Input: part model. Units: mm. Frame: model coordinates. A direction names the side the tool comes from. Give positions to 0.01 mm unless a question says otherwise; leave off trailing zeros. Loops run counter-clockwise (first coordinate to the right, second up) from the corner with the lowest first, then second, coordinate; pieces in that order, holes last. Notation, with made-up numbers: M 6,66 L 54,66 A24 cw 54,78 Z; hole C -13,45.5 d3. An arc over 180 degrees is marked long. Use a Markdown table: item, result. Add a question column.
from build123d import *

# Parameters (mm, degrees)
SKETCH_1_R      = 2.1
EXTRUDE_1_DEPTH = 17.45
SKETCH_2_R      = 4.15
EXTRUDE_2_DEPTH = 3.5
SKETCH_3_R      = 4.15
EXTRUDE_3_DEPTH = 3.5
FILLET_1_R      = 1.5


with BuildPart() as part:
    # ｽｹｯﾁ1 → ﾎﾞｽ - 押し出し1 (new body)
    with BuildSketch(Plane.XY):
        Polygon((-5, -13.5), (5, -13.5), (8.5, -10), (24.6, -10), (24.6, 10), (-24.6, 10), (-24.6, -10), (-8.5, -10), align=None)
        with Locations((-12.7, -4.3)):
            Circle(SKETCH_1_R, mode=Mode.SUBTRACT)
        with Locations(Location((12.7, -4.3, 0), (0, 0, 180))):
            Circle(SKETCH_1_R, mode=Mode.SUBTRACT)
    extrude(amount=EXTRUDE_1_DEPTH)

    # ｽｹｯﾁ2 → ﾎﾞｽ - 押し出し2 (add)
    with BuildSketch(Plane.XZ.offset(10)):
        with Locations(Location((-20, 8.725, 0), (0, 0, 180))):
            Circle(SKETCH_2_R)
        with Locations(Location((20, 8.725, 0), (0, 0, 180))):
            Circle(SKETCH_2_R)
    extrude(amount=EXTRUDE_2_DEPTH)

    # ｽｹｯﾁ3 → ﾎﾞｽ - 押し出し3 (add)
    with BuildSketch(Plane.XZ.offset(13.5)):
        with Locations(Location((0, 8.725, 0), (0, 0, 180))):
            Circle(SKETCH_3_R)
    extrude(amount=EXTRUDE_3_DEPTH)

    # ｽｹｯﾁ5 → 回転1 (revolve)
    with BuildSketch(Plane.XY.offset(8.725)):
        with BuildLine():
            Line((-10.6, 10), (-18.6, 10))
            Line((-18.6, 10), (-18.6, 12))
            Line((-18.6, 12), (-16.6, 12))
            Line((-16.6, 12), (-16.6, 25))
            Line((-16.6, 25), (-14.75, 25))
            Line((-14.75, 25), (-14.75, 31.78842818))
            ThreePointArc((-14.75, 31.78842818), (-15, 32.03842818), (-14.75, 32.28842818))
            Line((-14.75, 32.28842818), (-14.75, 34))
            ThreePointArc((-14.75, 34), (-12.680005458, 34.216234269), (-10.6, 34.28842818))
            Line((-10.6, 34.28842818), (-10.6, 34))
            Line((-10.6, 34), (-10.6, 10))
        make_face()
    revolve(axis=Axis((-10.6, 27.136449726, 8.725), (0, -1, 0)))

    # ﾌｨﾚｯﾄ1
    fillet_1_edges = [part.edges().sort_by_distance(p)[0] for p in [
        (24.6, 0, 17.45),
        (-24.6, 0, 17.45),
        (-24.6, 0, 0),
        (24.6, 0, 0),
    ]]
    fillet(fillet_1_edges, radius=FILLET_1_R)


solid = part.part
1) Contact query for flat-ended pins moving along their axis: P1, Ø1, axis at x = 13.5, z = 8, coming from the -Y side; P2, Ø6.5, axis at x = -21.5, z = 9, coming from the -Y side; P3, Ø3, axis at x = 8, z = 8, coming from the -Y side. Output: stop coordinate, or through.
2) Section query B-B, the plane y = -4.3. Return the cut outline in (x, z), and give its area (3 significant figures).
3) Ray query, line 1 (Y direction, x = -12.7, z = 4.25); line 2 (X direction, y = -12, z = 6.5); line 3 (X direction, y = -13, z = 7.5). Return the intervals inside material, ascending. Write a range as [from, to].
4) Reachability of faces 1 (the cylindrical face through (-6.454, 28.442, 8.543)), 2 (the flat face through (-20, -13.5, 9)), 3 (the flat face through (-14, 12, 3)) from +Z, -Z, +X, -X, +Y, -Y: full face, straight path, thin tool, end or side. Return the list, or none.
5) Section query D-D, the plane z = 14. Return the cut outline in (x, y).
6) Section query C-C, the plane x = -20. Return the cut outline in (y, z) (3 decimals), and give its area (3 significant figures).
7) Section query A-A, the plane x = 12.7. Return the cut outline in (y, z), and give its area (3 significant figures).
8) Pull-direction query (X, two-part tool) for faces 4 (the flat face through (6.7, -11.8, 8.6)), 5 (the flat face through (24.6, 0, 9)), 6 (the cylindrical face through (-9.819, 18.591, 2.776)); classes: pulls with the +X half, pulls with the -X half, needs draft (parallel to the pull), parting line crosses it, or undercut.
Entries:
| question | item | result |
|---|---|---|
| 1 | P1 | stops at y = -10 |
| 1 | P2 | stops at y = -13.5 |
| 1 | P3 | stops at y = -12 |
| 2 | outline | M -24.6,1.5 A1.5 ccw -23.1,0 L -14.8,0 L -14.8,17.45 L -23.1,17.45 A1.5 ccw -24.6,15.95 Z; M -10.6,0 L 10.6,0 L 10.6,17.45 L -10.6,17.45 Z; M 14.8,0 L 23.1,0 A1.5 ccw 24.6,1.5 L 24.6,15.95 A1.5 ccw 23.1,17.45 L 14.8,17.45 Z |
| 2 | area | 710 mm² |
| 3 | line 1 | y = [-10, -6.4], [-2.2, 25] |
| 3 | line 2 | x = [-23.5, -16.5], [-6.5, 6.5], [16.5, 23.5] |
| 3 | line 3 | x = [-23.97, -16.03], [-5.5, 5.5], [16.03, 23.97] |
| 4 | face 1 | none |
| 4 | face 2 | +Z, -Z, -X, -Y |
| 4 | face 3 | +Y |
| 5 | outline | M -24.6,-10 L -8.5,-10 L -5,-13.5 L 5,-13.5 L 8.5,-10 L 24.6,-10 L 24.6,10 L -4.59,10 L -4.59,12 L -7.74,12 L -7.74,25 L -13.46,25 L -13.46,12 L -16.61,12 L -16.61,10 L -24.6,10 Z; hole C -12.7,-4.3 d4.2; hole C 12.7,-4.3 d4.2 |
| 6 | outline | M -13.5,4.575 L -10,4.575 L -10,0 L 10,0 L 10,17.45 L -10,17.45 L -10,12.875 L -13.5,12.875 Z |
| 6 | area | 378 mm² |
| 7 | outline | M -10,0 L -6.4,0 L -6.4,17.45 L -10,17.45 Z; M -2.2,0 L 10,0 L 10,17.45 L -2.2,17.45 Z |
| 7 | area | 276 mm² |
| 8 | face 4 | undercut |
| 8 | face 5 | pulls with the +X half |
| 8 | face 6 | parting line crosses it |
